from build123d import *

# Parameters (mm, degrees)
SKETCH_1_R      = 3
SKETCH_1_R_2    = 1.5
EXTRUDE_1_DEPTH = 4


with BuildPart() as part:
    # 草图1 → 凸台-拉伸1 (new body)
    with BuildSketch(Plane.XY):
        with BuildLine():
            Line((1790.797367784, 1613.266845989), (1790.797367784, 1565.512011993))
            ThreePointArc((1790.797367784, 1565.512011993), (1788.297367784, 1558.012011993), (1790.797367784, 1550.512011993))
            Line((1790.797367784, 1550.512011993), (1790.797367784, 1502.757177997))
            ThreePointArc((1790.797367784, 1502.757177997), (1796.970533461, 1493.518382672), (1807.868435596, 1495.686110185))
            Line((1807.868435596, 1495.686110185), (1863.123269592, 1550.940944181))
            ThreePointArc((1863.123269592, 1550.940944181), (1866.05220178, 1558.012011993), (1863.123269592, 1565.083079805))
            Line((1863.123269592, 1565.083079805), (1807.868435596, 1620.337913801))
            ThreePointArc((1807.868435596, 1620.337913801), (1796.970533461, 1622.505641314), (1790.797367784, 1613.266845989))
        make_face()
        with Locations((1800.797367784, 1558.012011993)):
            Circle(SKETCH_1_R, mode=Mode.SUBTRACT)
        with Locations((1800.797367784, 1613.266845989)):
            Circle(SKETCH_1_R_2, mode=Mode.SUBTRACT)
        with Locations((1856.05220178, 1558.012011993)):
            Circle(SKETCH_1_R_2, mode=Mode.SUBTRACT)
        with Locations((1800.797367784, 1502.757177997)):
            Circle(SKETCH_1_R_2, mode=Mode.SUBTRACT)
        with BuildLine():
            ThreePointArc((1805.443255224, 1550.809308797), (1806.858027956, 1551.951351821), (1808.000070981, 1553.366124554))
            ThreePointArc((1808.000070981, 1553.366124554), (1807.55260939, 1555.43971519), (1805.479018754, 1554.992253599))
            ThreePointArc((1805.479018754, 1554.992253599), (1804.736707613, 1554.072672165), (1803.817126178, 1553.330361023))
            ThreePointArc((1803.817126178, 1553.330361023), (1803.369664588, 1551.256770387), (1805.443255224, 1550.809308797))
        make_face(mode=Mode.SUBTRACT)
        with BuildLine():
            ThreePointArc((1808.000070981, 1562.657899433), (1806.858027956, 1564.072672165), (1805.443255224, 1565.21471519))
            ThreePointArc((1805.443255224, 1565.21471519), (1803.369664588, 1564.767253599), (1803.817126178, 1562.693662963))
            ThreePointArc((1803.817126178, 1562.693662963), (1804.736707613, 1561.951351821), (1805.479018754, 1561.031770387))
            ThreePointArc((1805.479018754, 1561.031770387), (1807.55260939, 1560.584308797), (1808.000070981, 1562.657899433))
        make_face(mode=Mode.SUBTRACT)
        with BuildLine():
            ThreePointArc((1796.151480345, 1565.21471519), (1794.736707613, 1564.072672165), (1793.594664588, 1562.657899433))
            ThreePointArc((1793.594664588, 1562.657899433), (1794.042126178, 1560.584308797), (1796.115716814, 1561.031770387))
            ThreePointArc((1796.115716814, 1561.031770387), (1796.858027956, 1561.951351821), (1797.77760939, 1562.693662963))
            ThreePointArc((1797.77760939, 1562.693662963), (1798.225070981, 1564.767253599), (1796.151480345, 1565.21471519))
        make_face(mode=Mode.SUBTRACT)
        with BuildLine():
            ThreePointArc((1793.594664588, 1553.366124554), (1794.736707613, 1551.951351821), (1796.151480345, 1550.809308797))
            ThreePointArc((1796.151480345, 1550.809308797), (1798.225070981, 1551.256770387), (1797.77760939, 1553.330361023))
            ThreePointArc((1797.77760939, 1553.330361023), (1796.858027956, 1554.072672165), (1796.115716814, 1554.992253599))
            ThreePointArc((1796.115716814, 1554.992253599), (1794.042126178, 1555.43971519), (1793.594664588, 1553.366124554))
        make_face(mode=Mode.SUBTRACT)
    extrude(amount=EXTRUDE_1_DEPTH)


solid = part.part
Build history of the part. All positions in model axes, mm. A direction names the side the tool comes from. Round coordinates to 2 decimals unless told otherwise and drop trailing zeros. Loops run counter-clockwise (first coordinate to the right, second up) from the corner with the lowest first, then second, coordinate; pieces in that order, holes last. Notation, with made-up numbers: (79.25, 37) -> (123.25, 37) arc R18 cw to (123.25, 42) -> close; hole circle Ø6 at (18.25, 48.5). An arc over 180 degrees is marked (long way). Answer in a Markdown table with one row per item.
Item 1: Pin check, flat tips, straight feed: pin 1 (2.5 mm diameter, centred on x = 1800.8, y = 1502.76, fed in from +Z); pin 2 (2 mm diameter, centred on y = 1538.5, z = 2.5, fed in from -X); pin 3 (10 mm diameter, centred on x = 1828.5, y = 1560, fed in from -Z). Stop position of each tip, or through.
Answers below:
| item | result |
|---|---|
| pin 1 | passes through |
| pin 2 | stops at x = 1790.8 |
| pin 3 | stops at z = 0 |
Item 2: Which spindle directions (+Z, -Z, +X, -X, +Y, -Y) get a long thin tool onto all of the face, cutting with end or side? Do faces 4 (the flat face through (1790.797, 1590, 2)), 5 (the cylindrical face through (1794.72, 1551.97, 1.97)), 6 (the cylindrical face through (1797.123, 1622.567, 1.972)). Say none if no direction does.
Answers below:
| item | result |
|---|---|
| face 4 | +Z, -Z, -X, +Y |
| face 5 | +Z, -Z |
| face 6 | +Z, -Z, +Y |
Item 3: Drill centre lines: L1, parallel to X at y = 1564.5, z = 0.95; L2, parallel to Y at x = 1802, z = 3.15; L3, parallel to Y at x = 1807.5, z = 3.7. Where is each one in solid material? Low to high. Write a range as [from, to].
Answers below:
| item | result |
|---|---|
| L1 | x = [1790.11, 1795.2], [1798.36, 1803.23], [1806.4, 1863.66] |
| L2 | y = [1492.83, 1501.86], [1503.65, 1555.26], [1560.76, 1612.37], [1614.16, 1623.19] |
| L3 | y = [1495.34, 1552.67], [1555.47, 1560.55], [1563.35, 1620.69] |
Item 4: Saw through at A-A (x = 1856). Write the cut outline in (y, z).
Answers below:
| item | result |
|---|---|
| outline | (1543.82, 0) -> (1556.51, 0) -> (1556.51, 4) -> (1543.82, 4) -> close; (1559.51, 0) -> (1572.21, 0) -> (1572.21, 4) -> (1559.51, 4) -> close |
Item 5: Saw through at B-B (z = 2.55). State how many separate pieces and enclosed holes the cut face has, and give its area (3 significant figures).
Answers below:
| item | result |
|---|---|
| separate pieces | 1 |
| enclosed holes | 8 |
| area | 5,950 mm² |
Item 6: Saw through at C-C (y = 1530). Write the cut outline in (x, z), and give its area (3 significant figures).
Answers below:
| item | result |
|---|---|
| outline | (1790.8, 0) -> (1842.18, 0) -> (1842.18, 4) -> (1790.8, 4) -> close |
| area | 206 mm² |
Item 7: Saw through at D-D (x = 1834). Write the cut outline in (y, z), and give its area (3 significant figures).
Answers below:
| item | result |
|---|---|
| outline | (1521.82, 0) -> (1594.21, 0) -> (1594.21, 4) -> (1521.82, 4) -> close |
| area | 290 mm² |
Item 8: Mould opens along X. For faces 1 (the cylindrical face through (1798.207, 1551.229, 1.972)), 2 (the flat face through (1790.797, 1527, 2)), 3 (the flat face through (1835.883, 1592.324, 1.972)) say: +X half, -X half, draft (parallel to the pull), parting line (faces both ways), or undercut.
Answers below:
| item | result |
|---|---|
| face 1 | undercut |
| face 2 | -X half |
| face 3 | +X half |
